Source: three-view drawing plus pictorial views. Frame: mm from the lowest corner of the part. Round coordinates to 2 decimals unless told otherwise and drop trailing zeros. Order: outer loops, then holes, each group sorted by start corner. A loop starts at its lowest first (then second) coordinate and runs counter-clockwise, first axis right, second up. Notation, with made-up numbers: (77.5, 12.5) -> (132.5, 12.5) arc R23 ccw to (132.5, 47.5) -> close; hole circle Ø8 at (75.5, 69.25). An arc over 180 degrees is marked (long way). Answer as CSV lines item,"result".
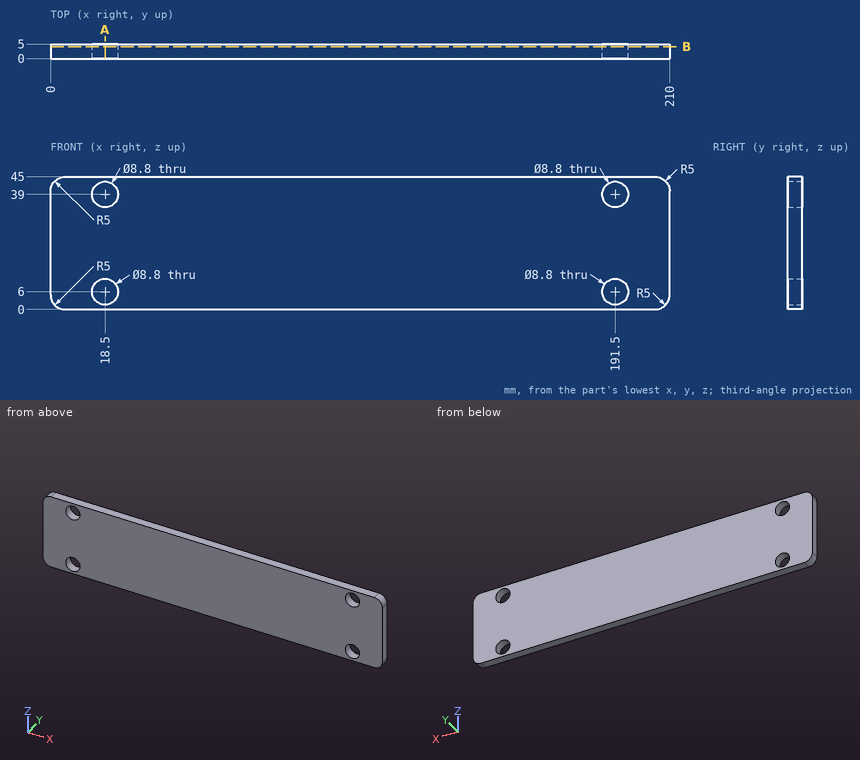
1. Section query B-B on y = 4.15. Return loops of the section in (x, z), and give its area (3 significant figures).
Results below:
outline,"(0, 5) arc R5 ccw to (5, 0) -> (205, 0) arc R5 ccw to (210, 5) -> (210, 40) arc R5 ccw to (205, 45) -> (5, 45) arc R5 ccw to (0, 40) -> close; hole circle Ø8.8 at (18.5, 6); hole circle Ø8.8 at (18.5, 39); hole circle Ø8.8 at (191.5, 6); hole circle Ø8.8 at (191.5, 39)"
area,"9,190 mm2"
2. Line query: L1, parallel to Z at x = 191.5, y = 2.65; L2, parallel to X at y = 3.6, z = 6.5; L3, parallel to X at y = 1.75, z = 40. Output: solid intervals per line, ascending. Write a range as [from, to].
Results below:
L1,"[0, 1.6], [10.4, 34.6], [43.4, 45]"
L2,"[0, 14.13], [22.87, 187.13], [195.87, 210]"
L3,"[0, 14.22], [22.78, 187.22], [195.78, 210]"
3. Pin query (flat end, axial travel): pin 1 (5 mm diameter, centred on x = 148, z = 29, fed in from -Y). Return the tip coordinate at first contact, or that it passes through.
Results below:
pin 1,"y = 0"
4. Section query A-A on x = 18.5. Return loops of the section in (y, z), and give its area (3 significant figures).
Results below:
outline,"(0, 0) -> (5, 0) -> (5, 1.6) -> (0, 1.6) -> close; (0, 10.4) -> (5, 10.4) -> (5, 34.6) -> (0, 34.6) -> close; (0, 43.4) -> (5, 43.4) -> (5, 45) -> (0, 45) -> close"
area,"137 mm2"
